Job drawing, mm, ordinate dimensions from the low corner. One solid piece. A direction names the side the tool comes from. Round coordinates to 2 decimals unless told otherwise and drop trailing zeros. Loops run counter-clockwise (first coordinate to the right, second up) from the corner with the lowest first, then second, coordinate; pieces in that order, holes last. Notation, with made-up numbers: (2, 82.5) - (35, 82.5) arc R8 cw to (35, 89.5) - close; hole circle Ø4 at (59.25, 44.25). An arc over 180 degrees is marked (long way). One line per question, with ' | ' between items. Start each with the question number.
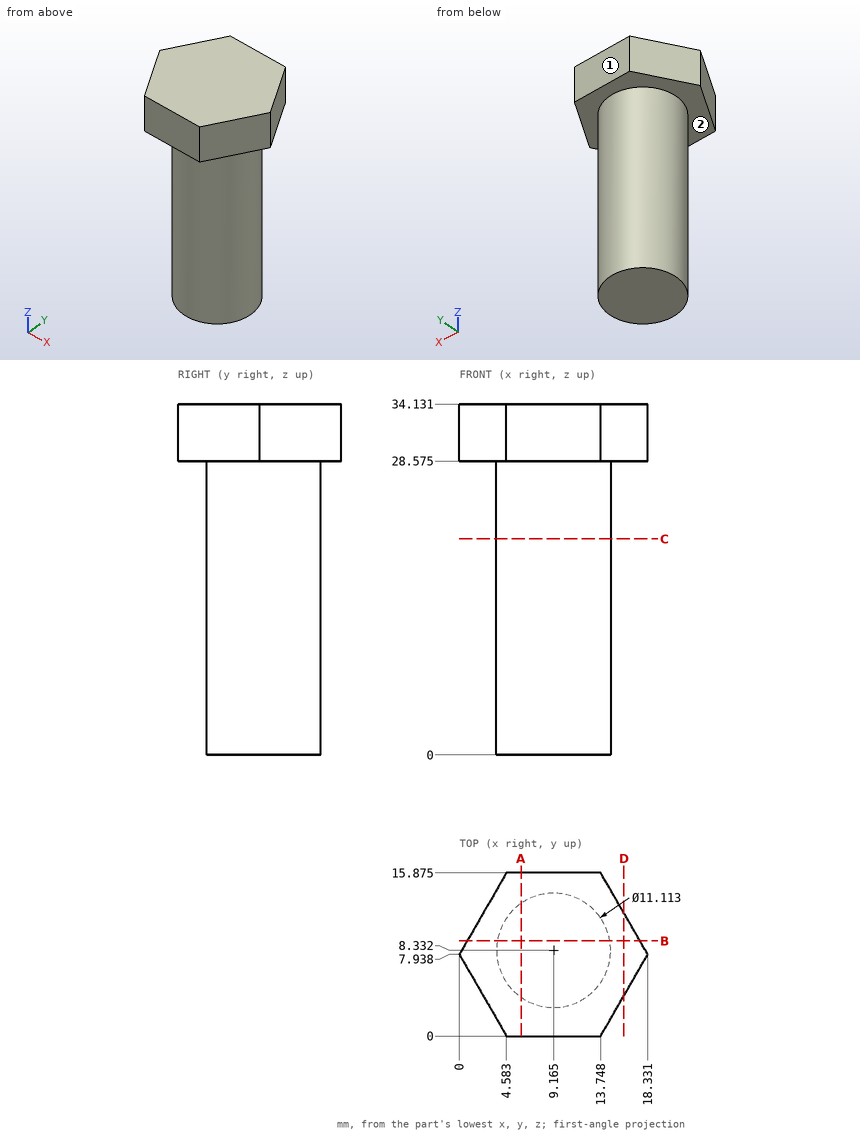
1) Wall check: line 1 (Z direction, x = 1.75, y = 5) (1 decimal); line 2 (X direction, y = 12.5, z = 5); line 3 (Y direction, x = 6, z = 13.5) (1 decimal). Give the ranges that are in metal, low to high. Write a range as [from, to].
2) Drop flat-ended pins along their axis: pin 1 (6 mm diameter, centred on x = 13.5, z = 20.5, fed in from -Y); pin 2 (6 mm diameter, centred on y = 5.5, z = 14, fed in from -X); pin 3 (6 mm diameter, centred on x = 16.5, z = 24.5, fed in from -Y) (1 decimal); pin 4 (4 mm diameter, centred on x = 11.5, y = 6, fed in from -Z). Give the stop position or say it passes through.
3) Tool access for the marked faces 1 and 2: list every direction of +Z, -Z, +X, -X, +Y, -Y with a clear straight run to the whole face (end or side of a thin tool).
4) Saw through at A-A on x = 6. Write the cut outline in (y, z) (1 decimal).
5) Saw through at C-C on z = 21. Write the cut outline in (x, y) (1 decimal), and give its area (3 significant figures).
6) Saw through at D-D on x = 16. Write the cut outline in (y, z) (1 decimal).
7) Saw through at B-B on y = 9.25. Write the cut outline in (x, z) (1 decimal), and give its area (3 significant figures).
Answer key:
1) line 1: [28.6, 34.1] | line 2: [5.49, 12.84] | line 3: [3.8, 12.9]
2) pin 1: y = 2.94 | pin 2: x = 3.61 | pin 3: y = 4.9 | pin 4: z = 0
3) face 1: +Z, -Z, +X, -X, +Y | face 2: -Z
4) outline: (0, 28.6) - (3.8, 28.6) - (3.8, 0) - (12.9, 0) - (12.9, 28.6) - (15.9, 28.6) - (15.9, 34.1) - (0, 34.1) - close
5) outline: circle Ø11.1 at (9.2, 8.3) | area: 97.0 mm²
6) outline: (3.9, 28.6) - (12, 28.6) - (12, 34.1) - (3.9, 34.1) - close
7) outline: (0.8, 28.6) - (3.7, 28.6) - (3.7, 0) - (14.6, 0) - (14.6, 28.6) - (17.6, 28.6) - (17.6, 34.1) - (0.8, 34.1) - close | area: 407 mm²
